Autodesk Inventor part; units mm, degrees
ref_plane "YZ Plane" through (0, 0, 0) normal (1, 0, 0) x (0, 1, 0)
ref_plane "XZ Plane" through (0, 0, 0) normal (0, 1, 0) x (-1, 0, 0)
ref_plane "XY Plane" through (0, 0, 0) normal (0, 0, 1) x (1, 0, 0)
sketch "Sketch1" plane through (0, 0, 0) normal (0, 1, 0) x (-1, 0, 0)
  line L0 (0, -37.4557) -> (0, 23.9689) construction
  line L1 (8, -2) -> (8, -12)
  line L2 (8, -12) -> (19, -12)
  line L3 (19, -12) -> (19, 12)
  line L4 (19, 12) -> (2, 12)
  line L5 (8, -2) -> (15, -2)
  line L6 (15, -2) -> (15, 3)
  line L7 (15, 3) -> (0, 3)
  line L8 (0, -49.7407) -> (0, 36.2538)
  line L9 (-8, -2) -> (-8, -12)
  line L10 (-8, -12) -> (-19, -12)
  line L11 (-19, -12) -> (-19, 12)
  line L12 (-19, 12) -> (2, 12)
  line L13 (-8, -2) -> (-15, -2)
  line L14 (-15, -2) -> (-15, 3)
  line L15 (-15, 3) -> (0, 3)
  line L16 (26.6, 0) -> (-26.6, 0)
  point P0 (19, 0)
  point P1 (-19, 0)
  dimension "d12" = 15
  dimension "d13" = 5
  dimension "d14" = 7
  dimension "d15" = 10
  dimension "d16" = 11
  dimension "d18" = 9
  dimension "d19" = 17
extrude "Extrusion1" add sketch "Sketch1" along normal blind 30 contours L5 L6 L16 L3 L2 L1 | L6 L7 L8 L12 L4 L3 L16 | L15 L14 L16 L11 L12 L8 | L14 L13 L9 L10 L11 L16
fillet "Fillet1" radius 4 2 edges at (-8, 15, -2) (8, 15, -2)
sketch "Sketch2" plane through (-19, 0, 12) normal (0, 0, 1) x (1, 0, 0)
  line L0 (0, 0) -> (38, 0)
  line L1 (38, 0) -> (38, 30)
  line L2 (0, 30) -> (38, 30)
  line L3 (0, 0) -> (0, 30)
  line L4 (38, 0) -> (38, 30)
  line L5 (38, 15) -> (0, 15) construction
  line L6 (0, 0) -> (0, 30)
  circle A0 centre (19, 15) radius 11
  circle A1 centre (19, 15) radius 5
  line L7 (0, 0) -> (38, 0)
  line L8 (7, 30) -> (7, 0)
  line L9 (4, 30) -> (7, 30)
  line L10 (4, 0) -> (4, 30)
  line L11 (4, 0) -> (7, 0)
  line L12 (31, 0) -> (31, 30)
  line L13 (31, 0) -> (34, 0)
  line L14 (34, 0) -> (34, 30)
  line L15 (31, 30) -> (34, 30)
  circle A2 centre (30.5, 27) radius 1.5
  line L16 (19, 15) -> (19, 38.5815) construction
  circle A3 centre (7.5, 27) radius 1.5
  circle A4 centre (30.5, 3) radius 1.5
  circle A5 centre (7.5, 3) radius 1.5
  point P0 (19, 0)
  dimension "d23" = 22
  dimension "d24" = 10
  dimension "d25" = 3
  dimension "d26" = 11.5
  dimension "d27" = 12
extrude "Extrusion2" cut sketch "Sketch2" against normal blind 7 contours A0
extrude "Extrusion3" cut sketch "Sketch2" against normal through all contours A5 L8 | L8 A5 | A4 L12 | L12 A4 | A3 L8 | L8 A3 | A2 L12 | L12 A2 | A1
fillet "Fillet2" radius 2 4 edges at (19, 15, 12) (-19, 15, 12) (-19, 15, -12) (19, 15, -12)
sketch "Boceto4" plane through (-17, 0, 12) normal (0, 0, 1) x (1, 0, 0)
  circle A0 centre (17, 15) radius 5
  line L0 (0, 0) -> (0, 30)
  line L1 (34, 30) -> (34, 0)
  line L2 (0, 0) -> (34, 0)
  line L3 (32, 30) -> (2, 30)
  line L4 (12, 30) -> (12, 24.798)
  circle A1 centre (17, 15) radius 11
  line L5 (22, 30) -> (22, 24.798)
  circle A2 centre (17, 15) radius 5 construction
  line L6 (17, 15) -> (17, 30) construction
  line L7 (32, 0) -> (2, 0) construction
  line L8 (12, 0) -> (12, 5.202)
  line L9 (22, 0) -> (22, 5.202)
  circle A3 centre (17, 15) radius 11
  line L10 (0, 30) -> (34, 30)
  circle A4 centre (5.5, 3) radius 1.5
  circle A5 centre (28.5, 27) radius 1.5
  circle A6 centre (5.5, 27) radius 1.5
  circle A7 centre (28.5, 3) radius 1.5
  line L11 (0, 0) -> (0, 30)
  line L12 (0, 0) -> (34, 0)
  line L13 (34, 30) -> (34, 0)
  line L14 (0, 30) -> (34, 30)
  circle A8 centre (17, 15) radius 11
  circle A9 centre (28.5, 27) radius 1.5
  circle A10 centre (5.5, 3) radius 1.5
  circle A11 centre (28.5, 3) radius 1.5
  point P0 (17, 0)
  dimension "d44" = 5
  dimension "d45" = 5
extrude "Extrusión5" cut sketch "Boceto4" against normal blind 2 contours L0 L10 L3 L4 A1 L8 L2 | L9 A1 L5 L3 L10 L1 L2
equation "\"d45\" = d44"
properties part number "Tensor" material "Plástico PBT"
The listing builds one solid part. Answer for the finished solid, in the listing's coordinates (mm). A direction names the side the tool comes from. Give positions to 0.01 mm unless a question says otherwise; leave off trailing zeros. Write each loop counter-clockwise with the first axis right and the second up, starting at its lowest first coordinate (ties: lowest second). Pieces come first, ordered by that corner, then holes. Notation, with made-up numbers: (-31.5, 31) -> (7.5, 31) arc R26 ccw to (7.5, 66) -> close; hole circle Ø5 at (-33.5, -33.5). An arc over 180 degrees is marked (long way). Write item = value, one per line. Start each with the question number.
1) The part is cut by section D-D, the plane y = 17.5. Determine the outline of the cut face in (x, z).
2) Straight lines are drawn through the part: line 1 along Y through (x, z) = (11.5, 7.5); line 2 along X through (y, z) = (3, -8); line 3 along Y through (x, z) = (0, 9). For each, find the intervals that lie inside material, in ascending order.
3) Each of these flat-tipped pins is pushed along its axis until it touches: pin 1 (1 mm diameter, centred on y = 2.5, z = 11, fed in from +X); pin 2 (8 mm diameter, centred on x = -3, y = 18, fed in from -Z); pin 3 (6 mm diameter, centred on x = -9.5, y = 18.5, fed in from +Z). Where does it stop, or does it pass through?
4) The part is cut by section A-A, the plane z = -6.5. Determine the outline of the cut face in (x, y), and give its area (3 significant figures).
5) The part is cut by section B-B, the plane x = 0. Determine the outline of the cut face in (y, z).
6) Determine the mould class of faces 4 (the face through (-5, 3, 11)), 5 (the face through (11.305, 28.487, 6.549)), 6 (the face through (0, 0, 6)), 7 (the face through (-11, 15, 8)) for opening direction Y: +Y half, -Y half, draft (parallel to the pull), parting line (faces both ways), or undercut.
7) The part is cut by section C-C, the plane z = 1.75. Determine the outline of the cut face in (x, y), and give its area (3 significant figures).
8) Which of the six approach directions +Z, -Z, +X, -X, +Y, -Y give full straight-line access (tool end or side, diameter ignored) to faces 1 (the face through (10.3, 2.1, 6.5)), 2 (the face through (15, 15, 0)), 3 (the face through (-17, 15, 11))?
Solutions:
q1.outline = (-19, -10) arc R2 ccw to (-17, -12) -> (-8, -12) -> (-8, -6) arc R4 ccw to (-12, -2) -> (-15, -2) -> (-15, 3) -> (-4.33, 3) -> (-4.33, 5) -> (-10.71, 5) -> (-10.71, 10) -> (-17, 10) -> (-17, 12) arc R2 ccw to (-19, 10) -> close; (4.33, 3) -> (15, 3) -> (15, -2) -> (12, -2) arc R4 ccw to (8, -6) -> (8, -12) -> (17, -12) arc R2 ccw to (19, -10) -> (19, 10) arc R2 ccw to (17, 12) -> (17, 10) -> (10.71, 10) -> (10.71, 5) -> (4.33, 5) -> close
q2.line_1 = 0 to 1.5, 4.5 to 25.5, 28.5 to 30
q2.line_2 = -19 to -13, -10 to -8, 8 to 10, 13 to 19
q2.line_3 = 0 to 4, 26 to 30
q3.pin_1 = 18.94
q3.pin_2 = 3
q3.pin_3 = 10
q4.outline = (-19, 0) -> (-8, 0) -> (-8, 30) -> (-19, 30) -> close; (8, 0) -> (19, 0) -> (19, 30) -> (8, 30) -> close; hole circle Ø3 at (-11.5, 3); hole circle Ø3 at (-11.5, 27); hole circle Ø3 at (11.5, 3); hole circle Ø3 at (11.5, 27)
q4.area = 632 mm²
q5.outline = (0, 3) -> (10, 3) -> (10, 5) -> (4, 5) -> (4, 12) -> (0, 12) -> close; (20, 3) -> (30, 3) -> (30, 12) -> (26, 12) -> (26, 5) -> (20, 5) -> close
q6.face_4 = draft
q6.face_5 = undercut
q6.face_6 = -Y half
q6.face_7 = undercut
q7.outline = (-19, 0) -> (-15, 0) -> (-15, 30) -> (-19, 30) -> close; (15, 0) -> (19, 0) -> (19, 30) -> (15, 30) -> close
q7.area = 240 mm²
q8.face_1 = +Z, -Z
q8.face_2 = +Y, -Y
q8.face_3 = +Z, +Y, -Y
